The listing builds one solid part. Answer for the finished solid, in the listing's coordinates (mm). A direction names the side the tool comes from. Round coordinates to 2 decimals unless told otherwise and drop trailing zeros. Write each loop counter-clockwise with the first axis right and the second up, starting at its lowest first coordinate (ties: lowest second). Pieces come first, ordered by that corner, then holes.
Item 1: Find the intervals of material crossed by probe 1 along X at (y, z) = (-13, 25.75); probe 2 along X at (y, z) = (-13.5, 23.75); probe 3 along Y at (x, z) = (8, 18.75), in increasing order.
Item 2: For a pull along X with two mould halves and no side action, classify faces 1 (the face through (17.38, -27.04, 14.36)), 2 (the face through (38.528, -12, 14)), 3 (the face through (45, -5.045, 14)), 4 (the face through (30.82, -16.19, 13.96)) as +X half, -X half, draft (parallel to the pull), parting line (faces both ways), or undercut.
Item 3: A tool of negligible diameter and unlimited length cuts with its end or side. For faces 5 (the face through (8, -5.045, 14)), 6 (the face through (35.676, -27.038, 14.358)), from which of +Z, -Z, +X, -X, +Y, -Y can it reach the whole face along a straight path? Write none if from no direction.
Item 4: Find section D-D on y = -7. Give the vertices of the cut face in (x, z).
Item 5: Each of these flat-tipped pins is pushed along its axis until it touches: pin 1 (5 mm diameter, centred on y = -12, z = 15.5, fed in from -X); pin 2 (10 mm diameter, centred on x = 21.5, z = 25, fed in from +Y); pin 3 (10.5 mm diameter, centred on x = 26.53, y = -17.54, fed in from -Z); pin 4 (4 mm diameter, centred on x = 5.5, z = 9.5, fed in from -Y). Where does it stop, or does it pass through?
Item 6: Find section A-A on y = -16. Give the vertices of the cut face in (x, z).
Item 7: Find section B-B on z = 21. Give the vertices of the cut face in (x, y).
Item 8: Find section C-C on x = 27. Give the vertices of the cut face in (y, z), then the cut area to 3 significant figures.
```python
from build123d import *

# Parameters (mm, degrees)
CROQUIS1_R              = 4.5
SALIENTE_EXTRUIR1_DEPTH = 28.32
REDONDEO1_R             = 10


with BuildPart() as part:
    # Croquis1 → Saliente-Extruir1 (new body)
    with BuildSketch(Plane.XY):
        Polygon((0.527798388, 0.005572044), (50.52777288, -0.044933007), (50.527798388, -5.044933007), (38.527798388, -5.044933007), (38.527798388, -30.044933007), (14.527798388, -30.044933007), (14.527798388, -5.044933007), (0.524677348, -5.044933007), align=None)
        with Locations((26.527798388, -17.544933007)):
            Circle(CROQUIS1_R, mode=Mode.SUBTRACT)
    extrude(amount=SALIENTE_EXTRUIR1_DEPTH)

    # Redondeo1
    redondeo1_edges = [part.edges().sort_by_distance(p)[0] for p in [
        (38.527798388, -30.044933007, 14.16),
        (14.527798388, -30.044933007, 14.16),
    ]]
    fillet(redondeo1_edges, radius=REDONDEO1_R)


solid = part.part
```
Check values:
1. probe 1: x = 14.53 to 38.53
1. probe 2: x = 14.53 to 24.56, 28.5 to 38.53
1. probe 3: y = -5.04 to 0
2. face 1: -X half
2. face 2: +X half
2. face 3: draft
2. face 4: undercut
3. face 5: +Z, -Z, -X, -Y
3. face 6: +Z, -Z, +X, -Y
4. outline: (14.53, 0) - (38.53, 0) - (38.53, 28.32) - (14.53, 28.32) - close
5. pin 1: stops at x = 14.53
5. pin 2: stops at y = -0.01
5. pin 3: stops at z = 0
5. pin 4: stops at y = -5.04
6. outline: (14.53, 0) - (22.3, 0) - (22.3, 28.32) - (14.53, 28.32) - close; (30.75, 0) - (38.53, 0) - (38.53, 28.32) - (30.75, 28.32) - close
7. outline: (0.52, -5.04) - (14.53, -5.04) - (14.53, -20.04) arc R10 ccw to (24.53, -30.04) - (28.53, -30.04) arc R10 ccw to (38.53, -20.04) - (38.53, -5.04) - (50.53, -5.04) - (50.53, -0.04) - (0.53, 0.01) - close; hole circle Ø9 at (26.53, -17.54)
8. outline: (-30.04, 0) - (-22.02, 0) - (-22.02, 28.32) - (-30.04, 28.32) - close; (-13.07, 0) - (-0.02, 0) - (-0.02, 28.32) - (-13.07, 28.32) - close
8. area: 597 mm2
